The model under review builds one solid part; all positions refer to its coordinate system, in mm. Face numbers are marked on the shaded views. A direction names the side the tool comes from. Coordinates: 2 decimals unless noted, no trailing zeros. Order: outer loops, then holes, each group sorted by start corner. A loop starts at its lowest first (then second) coordinate and runs counter-clockwise, first axis right, second up. Notation, with made-up numbers: M 10,37.25 L 35,37.25 A38 cw 35,76.25 Z; hole C 89,49 d8. An arc over 180 degrees is marked long. One line per item, written item: value.
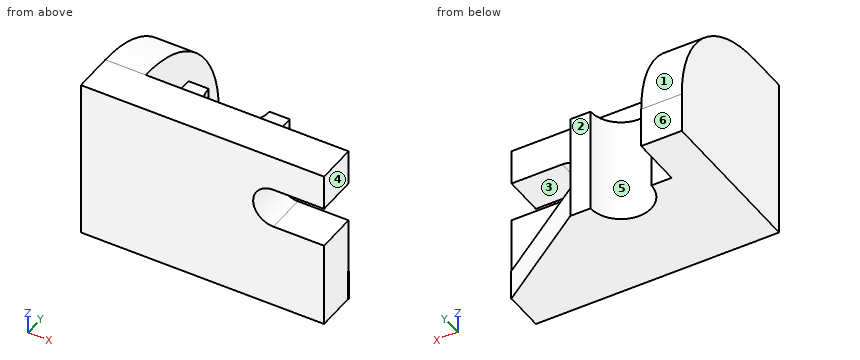
```python
from build123d import *

# Parameters (mm, degrees)
SKETCH1_W           = 96
SKETCH1_H           = 64
BOSS_EXTRUDE1_DEPTH = 16
CUT_EXTRUDE2_DEPTH  = 16
BOSS_EXTRUDE2_START = -22
BOSS_EXTRUDE2_DEPTH = 42
BOSS_EXTRUDE3_DEPTH = 16
BOSS_EXTRUDE4_DEPTH = 12


with BuildPart() as part:
    # Sketch1 → Boss-Extrude1 (new body)
    with BuildSketch(Plane(origin=(0, 0, 0), x_dir=(1, 0, 0), z_dir=(0, 1, 0))):
        Rectangle(SKETCH1_W, SKETCH1_H)
    extrude(amount=BOSS_EXTRUDE1_DEPTH)

    # Sketch2 → Cut-Extrude2 (cut)
    with BuildSketch(Plane(origin=(0, 16, 0), x_dir=(1, 0, 0), z_dir=(0, 1, 0))):
        with BuildLine():
            Line((48, -18), (28, -18))
            ThreePointArc((28, -18), (20, -10), (28, -2))
            Line((28, -2), (48, -2))
            ThreePointArc((48, -2), (56, -10), (48, -18))
        make_face()
    extrude(amount=-CUT_EXTRUDE2_DEPTH, mode=Mode.SUBTRACT)

    # Sketch3 → Boss-Extrude2 (add)
    with BuildSketch(Plane.XY.offset(32).offset(BOSS_EXTRUDE2_START)):
        with BuildLine():
            Line((-32, 44), (-32, 16))
            Line((-32, 16), (8, 16))
            Line((8, 16), (8, 44))
            Line((8, 44), (0, 44))
            ThreePointArc((0, 44), (-12, 32), (-24, 44))
            Line((-24, 44), (-32, 44))
        make_face()
    extrude(amount=-BOSS_EXTRUDE2_DEPTH)

    # Sketch5 → Boss-Extrude3 (add)
    with BuildSketch(Plane.ZY.offset(48)):
        with BuildLine():
            Line((-32, 0), (31.997051588, 0))
            Line((31.997051588, 0), (31.997051588, 16))
            ThreePointArc((31.997051588, 16), (17.938177085, 49.941125497), (-16.002948412, 64))
            Line((-16.002948412, 64), (-32, 64))
            Line((-32, 64), (-32, 0))
        make_face()
    extrude(amount=-BOSS_EXTRUDE3_DEPTH)

    # Sketch6 → Boss-Extrude4 (add)
    with BuildSketch(Plane(origin=(0, 0, -32), x_dir=(-1, 0, 0), z_dir=(0, 0, -1))):
        Polygon((-8, 44), (-48.368210029, 15.792048014), (-8, 16), align=None)
    extrude(amount=-BOSS_EXTRUDE4_DEPTH)


solid = part.part
```
(1) We need section A-A, the plane y = 14.5. State the section outline as (x, z) points.
Geometry results:
outline: M -48,-32 L 48,-32 L 48,2 L 28,2 A8 cw 28,18 L 48,18 L 48,32 L -48,32 Z
(2) We need section B-B, the plane x = -12. State the section outline as (y, z) points.
Geometry results:
outline: M 0,-32 L 32,-32 L 32,10 L 16,10 L 16,32 L 0,32 Z
(3) We need section C-C, the plane z = -26. State the section outline as (x, y) points.
Geometry results:
outline: M -48,0 L 48,0 L 48,15.79 L 48.37,15.79 L 8,44 L 0,44 A12 cw -24,44 L -32,44 L -32,64 L -48,64 Z
(4) Insertion check: pin 1 Ø6 at (x, y) = (18, 36.5) entering from +Z; pin 2 Ø4 at (y, z) = (23, 21) entering from +X; pin 3 Ø1.5 at (x, z) = (11, 23.5) entering from +Y. Each pin has a flat end and moves straight along its axis. Give the tip position at first contact, or say it passes through.
Geometry results:
pin 1: stops at z = -20
pin 2: stops at x = -32
pin 3: stops at y = 16
(5) For L1, parallel to Z at x = 21, y = 31; L2, parallel to Y at x = -29, z = -14.5; L3, parallel to X at y = 37.5, z = -25.5, list the stretches that pass through material, from the lowest coordinate up.
Geometry results:
L1: z = -32 to -20
L2: y = 0 to 44
L3: x = -48 to -22.09, -1.91 to 17.3
(6) We need section D-D, the plane x = 38. State the section outline as (y, z) points, plus the area to 3 significant figures.
Geometry results:
outline: M 0,-32 L 23.04,-32 L 23.04,-20 L 16,-20 L 16,2 L 0,2 Z; M 0,18 L 16,18 L 16,32 L 0,32 Z
area: 852 mm2
(7) Mouldability with a two-part tool opening along X and no side actions: class the marked faces 4, 5 and 6 as +X half, -X half, draft (parallel to the pull), parting line (faces both ways), or undercut.
Geometry results:
face 4: +X half
face 5: undercut
face 6: draft
(8) Tool access review of the marked faces 1, 2 and 3: name each direction out of +Z, -Z, +X, -X, +Y, -Y from which nothing blocks a thin tool from reaching the whole face with its end or side.
Geometry results:
face 1: +Z, +X, -X, +Y
face 2: +Z, -Z, +X, +Y
face 3: +X, +Y, -Y
